```python
from build123d import *

# Parameters (mm, degrees)
SKETCH1_W                 = 12.57
SKETCH1_H                 = 9.53
BOSS_EXTRUDE1_DEPTH       = 4
CUT_EXTRUDE1_REACH        = 14.57
CUT_EXTRUDE2_REACH        = 11.53
F_1_72_TAPPED_HOLE1_D     = 1.8288
F_1_72_TAPPED_HOLE1_DEPTH = 4


with BuildPart() as part:
    # Sketch1 → Boss-Extrude1 (new body)
    with BuildSketch(Plane.XY):
        Rectangle(SKETCH1_W, SKETCH1_H)
    extrude(amount=BOSS_EXTRUDE1_DEPTH)

    # Sketch2 → Cut-Extrude1 (cut, up to next)
    with BuildSketch(Plane.ZY.offset(6.285), mode=Mode.PRIVATE) as cut_extrude1_sk1:
        Polygon((4, 3.265), (4, -0.585), (2.075, 1.34), align=None)
    cut_extrude1_tool1 = extrude(cut_extrude1_sk1.sketch, amount=-CUT_EXTRUDE1_REACH, mode=Mode.PRIVATE) & part.part
    add(cut_extrude1_tool1.solids().sort_by_distance((-6.285, 1.34, 3.358333))[0], mode=Mode.SUBTRACT)

    # Sketch3 → Cut-Extrude2 (cut, up to next)
    with BuildSketch(Plane(origin=(0, 4.765, 0), x_dir=(1, 0, 0), z_dir=(0, 1, 0)), mode=Mode.PRIVATE) as cut_extrude2_sk1:
        Polygon((-2.221, -4), (-0.177343653, -1.956343653), (1.866312693, -4), align=None)
    cut_extrude2_tool1 = extrude(cut_extrude2_sk1.sketch, amount=-CUT_EXTRUDE2_REACH, mode=Mode.PRIVATE) & part.part
    add(cut_extrude2_tool1.solids().sort_by_distance((-0.177344, 4.765, 3.318781))[0], mode=Mode.SUBTRACT)

    # #1-72 Tapped Hole1
    with Locations(Plane.XY.offset(4)):
        with Locations((-4.253, -2.675), (4.075656347, -2.675)):
            Hole(F_1_72_TAPPED_HOLE1_D / 2, depth=F_1_72_TAPPED_HOLE1_DEPTH)


solid = part.part
```
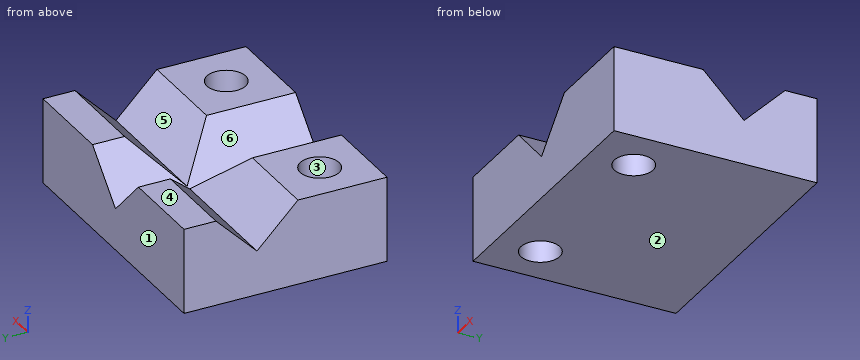
Input: part model. Units: mm. Frame: model coordinates. Face numbers are marked on the shaded views. A direction names the side the tool comes from. Give positions to 0.01 mm unless a question says otherwise; leave off trailing zeros. Order: outer loops, then holes, each group sorted by start corner. A loop starts at its lowest first (then second) coordinate and runs counter-clockwise, first axis right, second up. Notation, with made-up numbers: M 19,19 L 45,19 A16 ccw 45,46 Z; hole C 16,59 d2. An arc over 180 degrees is marked long. One line per question, with ' | ' between items. Start each with the question number.
1. Section query D-D (z = 3.1). Return the cut outline in (x, y) (3 decimals), and give its area (3 significant figures).
2. Pull-direction query (Y, two-part tool) for the marked faces 1, 2 and 3; classes: released by +Y, released by -Y, zero draft, split by the parting line, or undercut.
3. Section query A-A (z = 2.45). Return the cut outline in (x, y) (3 decimals), and give its area (3 significant figures).
4. Material intervals for probe 1 along X at (y, z) = (-2.75, 0.3) (3 decimals); probe 2 along X at (y, z) = (-3.5, 0.45) (3 decimals); probe 3 along Y at (x, z) = (-4.5, 2.65) (3 decimals), sorted ascending. Write a range as [from, to].
5. Section query B-B (x = 4.5). Return the cut outline in (y, z) (3 decimals), and give its area (3 significant figures).
6. Section query C-C (x = -2.75). Return the cut outline in (y, z) (3 decimals).
7. Access query for the marked faces 4, 5 and 6. Directions: +Z, -Z, +X, -X, +Y, -Y. A direction counts if a zero-diameter tool reaches every point of the face in a straight line with its end or side. Return the directions, or none.
Here are the results:
1) outline: M -6.285,-4.765 L -1.321,-4.765 L -1.321,0.315 L -6.285,0.315 Z; M -6.285,2.365 L -1.321,2.365 L -1.321,4.765 L -6.285,4.765 Z; M 0.966,-4.765 L 6.285,-4.765 L 6.285,0.315 L 0.966,0.315 Z; M 0.966,2.365 L 6.285,2.365 L 6.285,4.765 L 0.966,4.765 Z; hole C -4.253,-2.675 d1.829; hole C 4.076,-2.675 d1.829 | area: 71.7 mm²
2) face 1: released by +Y | face 2: zero draft | face 3: undercut
3) outline: M -6.285,-4.765 L -0.671,-4.765 L -0.671,0.965 L -6.285,0.965 Z; M -6.285,1.715 L -0.671,1.715 L -0.671,4.765 L -6.285,4.765 Z; M 0.316,-4.765 L 6.285,-4.765 L 6.285,0.965 L 0.316,0.965 Z; M 0.316,1.715 L 6.285,1.715 L 6.285,4.765 L 0.316,4.765 Z; hole C -4.253,-2.675 d1.829; hole C 4.076,-2.675 d1.829 | area: 96.4 mm²
4) probe 1: [-6.285, -5.164], [-3.342, 3.164], [4.987, 6.285] | probe 2: [-6.285, -4.647], [-3.859, 3.681], [4.47, 6.285] | probe 3: [-4.765, -3.555], [-1.795, 0.765], [1.915, 4.765]
5) outline: M -4.765,0 L -3.485,0 L -3.485,4 L -4.765,4 Z; M -1.865,0 L 4.765,0 L 4.765,4 L 3.265,4 L 1.34,2.075 L -0.585,4 L -1.865,4 Z | area: 27.9 mm²
6) outline: M -4.765,0 L 4.765,0 L 4.765,4 L 3.265,4 L 1.34,2.075 L -0.585,4 L -4.765,4 Z
7) face 4: +Z, +X, -X, +Y, -Y | face 5: +Z, +X, -X | face 6: +Z, +Y, -Y
